Answer from the drawing. Dimensions are ordinates in mm from the lowest x, y and z of the part. Coordinates: 2 decimals unless noted, no trailing zeros. Order: outer loops, then holes, each group sorted by start corner. A loop starts at its lowest first (then second) coordinate and runs counter-clockwise, first axis right, second up. Notation, with made-up numbers: (-15, -4) -> (12, -4) arc R26 ccw to (12, 20) -> close; hole circle Ø9 at (80.25, -10). An arc over 180 degrees is marked (long way). Answer as a JSON object with one key per item and string values. Group by question number.
1) Section B-B on z = 3 is taken. Determine the outline of the cut face in (x, y), and give its area (3 significant figures).
2) Consider L1, parallel to X at y = 1, z = 3; L2, parallel to Z at x = 3, y = 2.1; L3, parallel to X at y = 1.9, z = 40. Determine where each line is inside the solid, lowest interval first.
3) Section C-C on y = 2 is taken. Determine the outline of the cut face in (x, z), and give its area (3 significant figures).
4) Section A-A on x = 3 is taken. Determine the outline of the cut face in (y, z).
5) Given pin 1 (1.8 mm diameter, centred on x = 60, z = 3, fed in from +Y), flat-ended and moving along its own axis, determine where the tip first touches the part or whether it passes through.
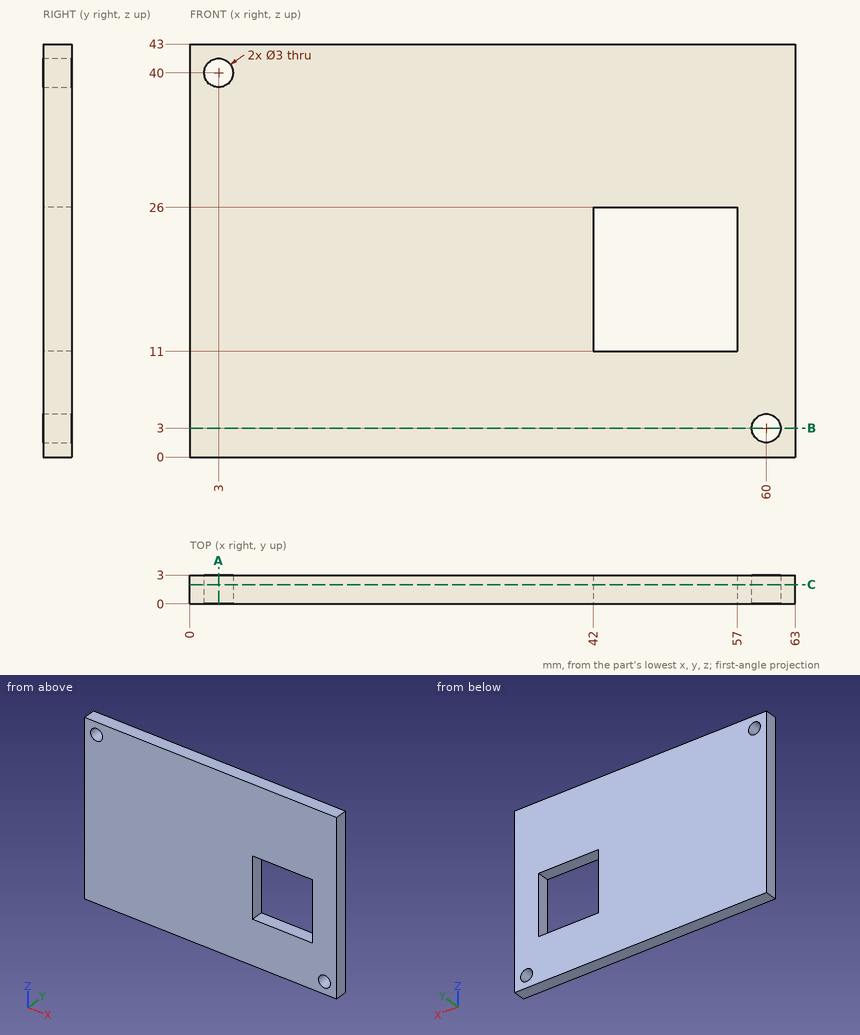
Worked answers:
{
 "1": {"outline": "(0, 0) -> (58.5, 0) -> (58.5, 3) -> (0, 3) -> close; (61.5, 0) -> (63, 0) -> (63, 3) -> (61.5, 3) -> close", "area": "180 mm²"},
 "2": {"L1": "x = 0 to 58.5, 61.5 to 63", "L2": "z = 0 to 38.5, 41.5 to 43", "L3": "x = 0 to 1.5, 4.5 to 63"},
 "3": {"outline": "(0, 0) -> (63, 0) -> (63, 43) -> (0, 43) -> close; hole circle Ø3 at (3, 40); hole (42, 11) -> (57, 11) -> (57, 26) -> (42, 26) -> close; hole circle Ø3 at (60, 3)", "area": "2,470 mm²"},
 "4": {"outline": "(0, 0) -> (3, 0) -> (3, 38.5) -> (0, 38.5) -> close; (0, 41.5) -> (3, 41.5) -> (3, 43) -> (0, 43) -> close"},
 "5": {"pin 1": "passes through"}
}
